Source: CAD feature listing. Evaluate the final solid. Frame: model axes, mm. A direction names the side the tool comes from. Give positions to 0.01 mm unless a question says otherwise; leave off trailing zeros. Order: outer loops, then holes, each group sorted by start corner. A loop starts at its lowest first (then second) coordinate and runs counter-clockwise, first axis right, second up. Notation, with made-up numbers: M -10,80 L 6,80 A14 cw 6,94 Z; hole C -37.5,36 d8. An arc over 180 degrees is marked long. Use CSV: the item, a comma, the result in double quotes. Start each with the question number.
Item 1: Section query B-B on y = 0.5. Return loops of the section in (x, z), and give its area (3 significant figures).
Item 2: Ray query, probe 1 along Y at (x, z) = (-6.5, 1); probe 2 along X at (y, z) = (-2.25, -4); probe 3 along Z at (x, y) = (-5.5, -3). Return the intervals inside material, ascending. Write a range as from..to.
Item 3: Pull-direction query (Z, two-part tool) for faces 1 (the face through (8, -5, 2)), 2 (the face through (-8.643, -2.465, -2.509)), 3 (the face through (3.31, -1.91, 6.43)); classes: +Z half, -Z half, draft (parallel to the pull), parting line (faces both ways), or undercut.
Item 4: Access query for faces 4 (the face through (7.226, -1.909, 0.348)), 5 (the face through (6.494, -2.465, -6.231)), 6 (the face through (-6.34, -1.91, 3.66)), 7 (the face through (8.643, -2.465, 2.509)), 8 (the face through (3.91, -1.91, -6.08)). Directions: +Z, -Z, +X, -X, +Y, -Y. A direction counts if a zero-diameter tool reaches every point of the face in a straight line with its end or side. Return the directions, or none.
Item 5: Section query A-A on y = -0.75. Count the separate pieces of the cut face and the enclosed holes in it, and give its area (3 significant figures).
Item 6: First-contact query: pin 1 (3 mm diameter, centred on x = 7.5, z = -2, fed in from -Y); pin 2 (5 mm diameter, centred on x = -5, y = 1, fed in from +Z); pin 3 (5 mm diameter, centred on x = -4, z = -0.5, fed in from -Y); pin 4 (5 mm diameter, centred on x = -4.5, z = -6.5, fed in from -Y). Flat tips, straight axial feed; report the tip coordinate or a pass-through.
from build123d import *

# Parameters (mm, degrees)
F2_DEPTH        = 5
F2_COPIES_COUNT = 6
F4_R            = 13.5
F5_DEPTH        = 4
F6_R            = 4.99999
F8_DEPTH        = 6
F10_DEPTH       = 1.5
F11_R           = 23.1793955011
F12_DEPTH       = 25


# Not quite as in the source:
# - a fillet or chamfer is up to 0.001 mm smaller than in the source, because OpenCascade refuses the exact size
# - a pattern or mirror of a feature is missing from the dataset's text; its kind, count and spacing are read off the source's solid


with BuildPart() as f2:
    # F1 (on Front) → F2 (new body)
    with BuildSketch(Plane.XZ):
        with BuildLine():
            Line((3.5710217678, 6.9345370094), (4.120409732, 8.001388857))
            ThreePointArc((4.120409732, 8.001388857), (2.1198467265, 8.7467851155), (0, 9))
            Line((0, 9), (0, 7.8))
            ThreePointArc((0, 7.8), (1.8372004963, 7.5805471001), (3.5710217678, 6.9345370094))
        make_face()
    extrude(amount=F2_DEPTH)


with BuildPart() as f2_copies_1:
    # F2_copies: instance of F2
    add(f2.part.rotate(Axis((0, 0, 0), (0, 1, 0)), 1 * 360 / F2_COPIES_COUNT))


with BuildPart() as f2_copies_2:
    # F2_copies: instance of F2
    add(f2.part.rotate(Axis((0, 0, 0), (0, 1, 0)), 2 * 360 / F2_COPIES_COUNT))


with BuildPart() as f2_copies_3:
    # F2_copies: instance of F2
    add(f2.part.rotate(Axis((0, 0, 0), (0, 1, 0)), 3 * 360 / F2_COPIES_COUNT))


with BuildPart() as f2_copies_4:
    # F2_copies: instance of F2
    add(f2.part.rotate(Axis((0, 0, 0), (0, 1, 0)), 4 * 360 / F2_COPIES_COUNT))


with BuildPart() as f2_copies_5:
    # F2_copies: instance of F2
    add(f2.part.rotate(Axis((0, 0, 0), (0, 1, 0)), 5 * 360 / F2_COPIES_COUNT))


with BuildPart() as f2_1:
    add(f2.part)

    add(f2_copies_1.part)  # F5 merges F2_copies_1

    add(f2_copies_2.part)  # F5 merges F2_copies_2

    add(f2_copies_3.part)  # F5 merges F2_copies_3

    add(f2_copies_4.part)  # F5 merges F2_copies_4

    add(f2_copies_5.part)  # F5 merges F2_copies_5
    # F4 (on Front) → F5 (join)
    with BuildSketch(Plane.XZ):
        with Locations((0, 3.5)):
            Circle(F4_R)
    extrude(amount=-F5_DEPTH)

    # F6 (radius 5 in the source; OpenCascade refuses exactly that, so slightly less here)
    f6_edges = [f2_1.edges().sort_by_distance(p)[0] for p in [
        (-1.8372, 0, -7.580547),
        (-7.483547, 0, -2.199211),
        (5.646346, 0, -5.381336),
        (-5.646346, 0, 5.381336),
        (7.483547, 0, 2.199211),
        (1.8372, 0, 7.580547),
    ]]
    fillet(f6_edges, radius=F6_R)

    # F7 (on face) → F8 (join)
    with BuildSketch(Plane.XZ):
        with BuildLine():
            ThreePointArc((-10, 0), (0, 10), (10, 0))
            Line((10, 0), (12, 0))
            ThreePointArc((12, 0), (0, 12), (-12, 0))
            Line((-12, 0), (-10, 0))
        make_face()
    extrude(amount=F8_DEPTH)

    # F9 (on face) → F10 (join)
    with BuildSketch(Plane.XZ.offset(6)):
        with BuildLine():
            Line((12, 0), (13.5, 0))
            ThreePointArc((13.5, 0), (0, 13.5), (-13.5, 0))
            Line((-13.5, 0), (-12, 0))
            ThreePointArc((-12, 0), (0, 12), (12, 0))
        make_face()
        with BuildLine():
            Line((10, 0), (12, 0))
            ThreePointArc((12, 0), (0, 12), (-12, 0))
            Line((-12, 0), (-10, 0))
            ThreePointArc((-10, 0), (0, 10), (10, 0))
        make_face()
    extrude(amount=F10_DEPTH)

    # F11 (on face) → F12 (cut)
    with BuildSketch(Plane(origin=(0, 4, 0), x_dir=(-1, 0, 0), z_dir=(0, 1, 0))):
        Circle(F11_R)
        with BuildLine():
            ThreePointArc((13.5, 3.5), (9.5459415677, -6.0459415243), (6.13e-08, -10))
            ThreePointArc((6.13e-08, -10), (-9.5459415677, 13.0459415243), (13.5, 3.5))
        make_face(mode=Mode.SUBTRACT)
        with BuildLine():
            ThreePointArc((13.5, 3.5), (-9.5459415677, 13.0459415243), (6.13e-08, -10))
            ThreePointArc((6.13e-08, -10), (9.5459415677, -6.0459415243), (13.5, 3.5))
        make_face()
        with BuildLine():
            ThreePointArc((6.13e-08, -10), (-7.0710678335, 7.0710677902), (10, 0))
            ThreePointArc((10, 0), (7.0710678335, -7.0710677902), (6.13e-08, -10))
        make_face(mode=Mode.SUBTRACT)
    extrude(amount=-F12_DEPTH, mode=Mode.SUBTRACT)


solid = f2_1.part
Verdict:
1,outline,"C 0,0 d20"
1,area,"314 mm2"
2,probe 1,"0..4"
2,probe 2,"-8.06..-6.93, 5.72..6.93"
2,probe 3,"4.92..7.12"
3,face 1,"draft"
3,face 2,"-Z half"
3,face 3,"undercut"
4,face 4,"+X, -Y"
4,face 5,"-Z, +X, -Y"
4,face 6,"-X, -Y"
4,face 7,"+Z, +X, -Y"
4,face 8,"-Z, -Y"
5,separate pieces,"6"
5,enclosed holes,"0"
5,area,"73.4 mm2"
6,pin 1,"y = 0"
6,pin 2,"z = 9.68"
6,pin 3,"y = -1.67"
6,pin 4,"y = -5"
